Autodesk Inventor part; units mm, degrees
ref_plane "Arbeitsebene1" through (0, 10, 0) normal (0, 1, 0) x (1, 0, 0)
ref_plane "YZ Plane" through (0, 0, 0) normal (1, 0, 0) x (0, 1, 0)
ref_plane "XZ Plane" through (0, 0, 0) normal (0, 1, 0) x (-1, 0, 0)
sketch "Skizze1" plane through (0, 0, 0) normal (0, 0, 1) x (1, 0, 0)
  line L0 (0, 0) -> (36.5, 0)
  line L1 (36.5, 0) -> (36.5, 20)
  line L2 (36.5, 20) -> (0, 20)
  line L3 (0, 20) -> (0, 0)
  dimension "d0" = 36.5
  dimension "d1" = 20
extrude "Extrusion1" add sketch "Skizze1" along normal blind 13.7
ref_plane "Arbeitsebene1" through (0, 10, 0) normal (0, 1, 0) x (1, 0, 0)
fillet "Rundung1" radius 10 2 edges at (36.5, 20, 6.85) (36.5, 0, 6.85)
sketch "Skizze2" plane through (0, 0, 0) normal (0, 0, -1) x (-1, 0, 0)
  arc A0 (-26.5, 20) -> (-26.5, 0) centre (-26.5, 10) ccw
  circle A1 centre (-27, 10) radius 2.5
  circle A2 centre (-27, 10) radius 1.5
  dimension "d5" = 5
  dimension "d6" = 10
  dimension "d7" = 12
  dimension "d8" = 3
extrude "Extrusion2" add sketch "Skizze2" along normal blind 0.3
sketch "Skizze4" plane through (0, 0, 0) normal (0, 0, -1) x (-1, 0, 0)
  line L0 (0, 0) -> (-26.5, 0)
  line L1 (0, 20) -> (0, 0)
  circle A0 centre (-19.65, 2.15) radius 1.15
  dimension "d15" = 2.3
  dimension "d16" = 1
  dimension "d17" = 18.5
extrude "Extrusion4" cut sketch "Skizze4" against normal through all
sketch "Skizze5" plane through (0, 0, 0) normal (0, 0, -1) x (-1, 0, 0)
  line L0 (0, 0) -> (-26.5, 0)
  line L1 (0, 20) -> (0, 0)
  circle A0 centre (-11, 6.5) radius 1.5
  dimension "d21" = 3
  dimension "d23" = 5
  dimension "d24" = 9.5
extrude "Extrusion8" add sketch "Skizze5" along normal blind 0.53
sketch "Skizze6" plane through (0, 0, 0) normal (0, 0, -1) x (-1, 0, 0)
  line L0 (0, 20) -> (0, 0)
  line L1 (-26.5, 20) -> (0, 20)
  circle A0 centre (-17.6, 11.9) radius 1.5
  dimension "d27" = 3
  dimension "d28" = 6.6
  dimension "d29" = 16.1
extrude "Extrusion5" add sketch "Skizze6" along normal up to surface (0.3 mm away)
sketch "Skizze7" plane through (0, 0, 13.7) normal (0, 0, 1) x (1, 0, 0)
  line L0 (0, 20) -> (0, 0)
  line L1 (0, 0) -> (26.5, 0)
  circle A0 centre (27, 10) radius 2.5
  circle A1 centre (27, 10) radius 3.65
  circle A2 centre (17.7, 11.6) radius 1.5
  dimension "d34" = 7.3
  dimension "d40" = 3
  dimension "d42" = 10.1
  dimension "d43" = 19.2
extrude "Extrusion9" add sketch "Skizze7" along normal blind 0.2
sketch "Skizze8" plane through (27, 10, 13.7) normal (0, 0, 1) x (1, 0, 0)
  circle A0 centre (0, 0) radius 2.5
  point P0 (-27, -10)
extrude "Extrusion10" add sketch "Skizze8" along normal blind 0.3
sketch "Skizze11" plane through (0, 20, 13.7) normal (0, 1, 0) x (1, 0, 0)
  line L0 (0, 13.7) -> (0, 0)
  line L1 (26.5, 0) -> (0, 0)
  line L2 (1, 0) -> (10.5, 0)
  line L3 (10.5, 0) -> (10.5, 2.8)
  line L4 (10.5, 2.8) -> (1, 2.8)
  line L5 (1, 2.8) -> (1, 0)
  dimension "d49" = 9.5
  dimension "d50" = 2.8
  dimension "d51" = 1
extrude "Extrusion11" add sketch "Skizze11" along normal blind 2.35
sketch "Skizze12" plane through (10.5, 20, 10.9) normal (0, 0, -1) x (-1, 0, 0)
  line L0 (9.5, 0) -> (0, 0)
  line L1 (9.5, 0) -> (9.5, 2.35)
  line L2 (0, 2.35) -> (9.5, 2.35)
  line L3 (0, 0) -> (0, 2.35)
  line L4 (1, 1.35) -> (8.5, 1.35)
  line L5 (8.5, 1.35) -> (8.5, 0)
  line L6 (8.5, 0) -> (1, 0)
  line L7 (1, 0) -> (1, 1.35)
  point P0 (10.5, -20)
  dimension "d54" = 1
  dimension "d55" = 1
  dimension "d56" = 1
extrude "Extrusion12" cut sketch "Skizze12" against normal through all contours L0 L7 L4 L5
mirror "Spiegeln1" about plane through (0, 10, 0) normal (0, 1, 0) of "Extrusion12", "Extrusion11"
properties part number "front"
Here's how the part is built. I have some questions about the finished solid (model axes, mm). A direction names the side the tool comes from. Round coordinates to 2 decimals unless told otherwise and drop trailing zeros. Loops run counter-clockwise (first coordinate to the right, second up) from the corner with the lowest first, then second, coordinate; pieces in that order, holes last. Notation, with made-up numbers: (-6.5, 56.5) - (28.5, 56.5) arc R29 cw to (28.5, 82.5) - close; hole circle Ø9 at (63, -10). An arc over 180 degrees is marked (long way). One line per question, with ' | ' between items. Start each with the question number.
Q1. We'd pull the mould along X, two halves only. Please class faces 1 (the cylindrical face through (33.65, 16.99, 6.95)), 2 (the flat face through (18, 12, -0.3)), 3 (the flat face through (2, 21, 12)), 4 (the flat face through (6, -1.35, 12)): +X half, -X half, draft (parallel to the pull), parting line (faces both ways), or undercut.
Q2. I want a section at C-C (y = 20.75). Write out the boundary of the cut face in (x, z).
Q3. Will these pins go through, and if not, where does the flat tip stop? pin 1 (4 mm diameter, centred on y = 11, z = 6, fed in from +X); pin 2 (1.5 mm diameter, centred on x = 26.5, y = 10.5, fed in from -Z); pin 3 (0.7 mm diameter, centred on y = -0.5, z = 12.5, fed in from -X); pin 4 (3 mm diameter, centred on y = 17.5, z = 4, fed in from +X).
Q4. I want a section at A-A (z = 12.25). State how many separate pieces and enclosed holes the cut face has, then the cut area to 3 significant figures.
Q5. Please list where these lines run through material, in increasing order: line 1 (Y direction, x = 19.65, z = 7.25); line 2 (Y direction, x = 27, z = -0.15); line 3 (Y direction, x = 7.5, z = 11.5). Write a range as [from, to].
Q6. For faces 5 (the flat face through (27, 10, 14)), 6 (the flat face through (2, -1, 12)), 7 (the flat face through (6, 22, 10.9)), 8 (the flat face through (29, 8, 13.9)), 9 (the flat face through (1, -1, 12)), which set-ups out of +Z, -Z, +X, -X, +Y, -Y let a thin tool reach every point of the face, with its end or its side?
Q7. I want a section at B-B (x = 7). Write out the boundary of the cut face in (y, z).
Response values:
1) face 1: +X half | face 2: draft | face 3: undercut | face 4: undercut
2) outline: (1, 10.9) - (2, 10.9) - (2, 13.7) - (1, 13.7) - close; (9.5, 10.9) - (10.5, 10.9) - (10.5, 13.7) - (9.5, 13.7) - close
3) pin 1: stops at x = 36.5 | pin 2: stops at z = 0 | pin 3: stops at x = 1 | pin 4: stops at x = 34.5
4) separate pieces: 1 | enclosed holes: 3 | area: 707 mm²
5) line 1: y = [0, 1], [3.3, 20] | line 2: y = [7.5, 8.5], [11.5, 12.5] | line 3: y = [-2.35, -1.35], [0, 20], [21.35, 22.35]
6) face 5: +Z, +X, -X, +Y, -Y | face 6: +Z, -Z | face 7: -Z, +X, -X, +Y | face 8: +Z | face 9: +Z, -Z, -X, -Y
7) outline: (-2.35, 10.9) - (-1.35, 10.9) - (-1.35, 13.7) - (-2.35, 13.7) - close; (0, 0) - (20, 0) - (20, 13.7) - (0, 13.7) - close; (21.35, 10.9) - (22.35, 10.9) - (22.35, 13.7) - (21.35, 13.7) - close
